```python
from build123d import *

# Parameters (mm, degrees)
F1_DEPTH = 0.4
F0_W     = 2
F0_H     = 2
F2_DEPTH = 8


with BuildPart() as f1:
    # F0 (on Front) → F1 (new body)
    with BuildSketch(Plane.XZ):
        Polygon((12.375, 5.125), (12.375, 7.125), (-12.375, 7.125), (-12.375, 5.125), (-14.375, 5.125), (-14.375, -5.125), (-12.375, -5.125), (-12.375, -7.125), (12.375, -7.125), (12.375, -5.125), (14.375, -5.125), (14.375, 5.125), align=None)
    extrude(amount=F1_DEPTH)

    # F0 (on Front) → F2 (join)
    with BuildSketch(Plane.XZ):
        with Locations((-13.375, 6.125)):
            Rectangle(F0_W, F0_H)
        with Locations((-13.375, -6.125)):
            Rectangle(F0_W, F0_H)
        with Locations((13.375, -6.125)):
            Rectangle(F0_W, F0_H)
        with Locations((13.375, 6.125)):
            Rectangle(F0_W, F0_H)
    extrude(amount=F2_DEPTH)


solid = f1.part
```
For this review, take the finished solid that the model builds, in its own axes (mm). A direction names the side the tool comes from. Round coordinates to 2 decimals unless told otherwise and drop trailing zeros. Loops run counter-clockwise (first coordinate to the right, second up) from the corner with the lowest first, then second, coordinate; pieces in that order, holes last.
Q1. Mouldability with a two-part tool opening along X and no side actions: class faces 4 (the face through (-12.375, -4, 6)), 5 (the face through (-13, -8, 6)) as +X half, -X half, draft (parallel to the pull), parting line (faces both ways), or undercut.
Result sheet:
face 4: undercut
face 5: draft
Q2. Machinability: for faces 1 (the face through (13, -8, -6)), 2 (the face through (12.375, -4, -6)), 3 (the face through (-13, -4, -5.125)), which of the approach directions +Z, -Z, +X, -X, +Y, -Y give a long, thin tool a straight path to every point of the face, cutting with its end or side? Answer none if there is none.
Result sheet:
face 1: +Z, -Z, +X, -X, -Y
face 2: +Z, -Z, -Y
face 3: +X, -X, -Y
Q3. Insertion check: pin 1 Ø4.5 at (x, z) = (7, -2) entering from -Y; pin 2 Ø1.5 at (x, y) = (0.5, -1.5) entering from -Z. Each pin has a flat end and moves straight along its axis. Give the tip position at first contact, or say it passes through.
Result sheet:
pin 1: stops at y = -0.4
pin 2: passes through
Q4. To check wall thickness, follow line 1 along X through (y, z) = (-4.75, 5.25) (3 decimals); line 2 along Y through (x, z) = (5.25, 0.75). State the ranges of each line that lie inside material, in increasing order.
Result sheet:
line 1: x = -14.375 to -12.375, 12.375 to 14.375
line 2: y = -0.4 to 0
Q5. Add section B-B on x = 6. Write out the cut boundary in (y, z) (3 decimals).
Result sheet:
outline: (-0.4, -7.125) - (0, -7.125) - (0, 7.125) - (-0.4, 7.125) - close
Q6. Add section C-C on z = -0.25. Write out the cut boundary in (x, y) (3 decimals), plus the area to 3 significant figures.
Result sheet:
outline: (-14.375, -0.4) - (14.375, -0.4) - (14.375, 0) - (-14.375, 0) - close
area: 11.5 mm2
Q7. Add section A-A on y = -3.75. Write out the cut boundary in (x, z) (3 decimals).
Result sheet:
outline: (-14.375, -7.125) - (-12.375, -7.125) - (-12.375, -5.125) - (-14.375, -5.125) - close; (-14.375, 5.125) - (-12.375, 5.125) - (-12.375, 7.125) - (-14.375, 7.125) - close; (12.375, -7.125) - (14.375, -7.125) - (14.375, -5.125) - (12.375, -5.125) - close; (12.375, 5.125) - (14.375, 5.125) - (14.375, 7.125) - (12.375, 7.125) - close
